```python
from build123d import *

# Parameters (mm, degrees)
SKETCH1_R           = 1.5
BOSS_EXTRUDE1_DEPTH = 6.35
SKETCH2_R           = 1.35255
CUT_EXTRUDE1_DEPTH  = 15.4526
FILLET1_R           = 3.175


with BuildPart() as part:
    # Sketch1 → Boss-Extrude1 (new body)
    with BuildSketch(Plane.XY):
        Polygon((0, 0), (15.875, 0), (15.875, 14.4526), (9.525, 14.4526), (9.525, 10.414), (0, 10.414), align=None)
        with Locations((11.43, 4.064)):
            Circle(SKETCH1_R, mode=Mode.SUBTRACT)
    boss_extrude1 = extrude(amount=BOSS_EXTRUDE1_DEPTH)

    # Mirror1: Boss-Extrude1 across plane
    add(boss_extrude1.mirror(Plane(origin=(0, 10.414, 6.35), x_dir=(0, 0, 1), z_dir=(1, 0, 0))))

    # Sketch2 → Cut-Extrude1 (cut, through all)
    with BuildSketch(Plane.XZ):
        with Locations((0, 3.175)):
            Circle(SKETCH2_R)
    extrude(amount=-CUT_EXTRUDE1_DEPTH, mode=Mode.SUBTRACT)

    # Fillet1
    fillet1_edges = [part.edges().sort_by_distance(p)[0] for p in [
        (15.875, 0, 3.175),
        (-15.875, 0, 3.175),
    ]]
    fillet(fillet1_edges, radius=FILLET1_R)


solid = part.part
```
Could you check a few things on this model? Use its own coordinates, in mm. A direction names the side the tool comes from. Round coordinates to 2 decimals unless told otherwise and drop trailing zeros. Loops run counter-clockwise (first coordinate to the right, second up) from the corner with the lowest first, then second, coordinate; pieces in that order, holes last. Notation, with made-up numbers: (-36.5, -5.75) -> (15.5, -5.75) arc R9 cw to (15.5, 0.25) -> close; hole circle Ø11 at (67.25, -37.5). An arc over 180 degrees is marked (long way). One line per question, with ' | ' between items.
(1) If we section it at C-C on z = 4: List the corners of the cut face in (x, y) for me (3 decimals).
Model answer:
outline: (-15.875, 3.175) arc R3.175 ccw to (-12.7, 0) -> (-1.072, 0) -> (-1.072, 10.414) -> (-9.525, 10.414) -> (-9.525, 14.453) -> (-15.875, 14.453) -> close; (1.072, 0) -> (12.7, 0) arc R3.175 ccw to (15.875, 3.175) -> (15.875, 14.453) -> (9.525, 14.453) -> (9.525, 10.414) -> (1.072, 10.414) -> close; hole circle Ø3 at (-11.43, 4.064); hole circle Ø3 at (11.43, 4.064)
(2) If we section it at A-A on y = 13.5: List the corners of the cut face in (x, z) for me (3 decimals), and give its area (3 significant figures).
Model answer:
outline: (-15.875, 0) -> (-9.525, 0) -> (-9.525, 6.35) -> (-15.875, 6.35) -> close; (9.525, 0) -> (15.875, 0) -> (15.875, 6.35) -> (9.525, 6.35) -> close | area: 80.6 mm^2
(3) If we section it at B-B on x = -11.43: List the corners of the cut face in (y, z) for me.
Model answer:
outline: (0, 0) -> (2.56, 0) -> (2.56, 6.35) -> (0, 6.35) -> close; (5.56, 0) -> (14.45, 0) -> (14.45, 6.35) -> (5.56, 6.35) -> close
(4) For pin 1 Ø3 at (x, z) = (-3.5, 2) entering from +Y, with a flat end and sliding along its axis, tell me the tip position at first contact or that it passes through.
Model answer:
pin 1: stops at y = 10.41
(5) If we section it at D-D on z = 0.5: List the corners of the cut face in (x, y) for me (3 decimals).
Model answer:
outline: (-15.875, 3.175) arc R3.175 ccw to (-12.7, 0) -> (12.7, 0) arc R3.175 ccw to (15.875, 3.175) -> (15.875, 14.453) -> (9.525, 14.453) -> (9.525, 10.414) -> (-9.525, 10.414) -> (-9.525, 14.453) -> (-15.875, 14.453) -> close; hole circle Ø3 at (-11.43, 4.064); hole circle Ø3 at (11.43, 4.064)
(6) For faces 4 (the face through (0, 0, 5)), 5 (the face through (0, 10.414, 5)), which set-ups out of +Z, -Z, +X, -X, +Y, -Y let a thin tool reach every point of the face, with its end or its side?
Model answer:
face 4: +Z, -Z, +X, -X, -Y | face 5: +Z, -Z, +Y
(7) Thinking about a two-plate mould opening in Z: for faces 1 (the face through (0, 6, 6.35)), 2 (the face through (0.727, 5.134, 4.315)), 3 (the face through (-13, 14.453, 3)), which applies, released by +Z, released by -Z, zero draft, split by the parting line, or undercut?
Model answer:
face 1: released by +Z | face 2: undercut | face 3: zero draft
(8) If I drill on probe 1 along X at (y, z) = (3, 2.5); probe 2 along Z at (x, y) = (0, 3); probe 3 along Y at (x, z) = (11.43, 4.75), over which ranges is the centre line in solid material (lowest first)?
Model answer:
probe 1: x = -15.87 to -12.49, -10.37 to -1.17, 1.17 to 10.37, 12.49 to 15.87 | probe 2: z = 0 to 1.82, 4.53 to 6.35 | probe 3: y = 0 to 2.56, 5.56 to 14.45
